```python
from build123d import *

# Parameters (mm, degrees)
SKETCH1_R           = 25.4
SKETCH1_R_2         = 19.05
BOSS_EXTRUDE1_DEPTH = 50.8
SKETCH4_R           = 25.4
SKETCH4_R_2         = 23.8125
CUT_EXTRUDE1_DEPTH  = 1.5875
FILLET1_R           = 0.762


with BuildPart() as part:
    # Sketch1 → Boss-Extrude1 (new body)
    with BuildSketch(Plane.XY):
        Circle(SKETCH1_R)
        Circle(SKETCH1_R_2, mode=Mode.SUBTRACT)
    extrude(amount=BOSS_EXTRUDE1_DEPTH)

    # Sketch4 → Cut-Extrude1 (cut)
    with BuildSketch(Plane(origin=(0, 0, 0), x_dir=(-1, 0, 0), z_dir=(0, 0, -1))):
        Circle(SKETCH4_R)
        Circle(SKETCH4_R_2, mode=Mode.SUBTRACT)
    cut_extrude1 = extrude(amount=-CUT_EXTRUDE1_DEPTH, mode=Mode.SUBTRACT)

    # Mirror1: Cut-Extrude1 across plane
    add(cut_extrude1.mirror(Plane.XY.offset(25.4)), mode=Mode.SUBTRACT)

    # Fillet1
    fillet1_edges = [part.edges().sort_by_distance(p)[0] for p in [
        (23.8125, 0, 1.5875),
        (23.8125, 0, 49.2125),
    ]]
    fillet(fillet1_edges, radius=FILLET1_R)


solid = part.part
```
Verification items for the finished model (mm, model axes). A direction names the side the tool comes from. Round coordinates to 2 decimals unless told otherwise and drop trailing zeros. Write each loop counter-clockwise with the first axis right and the second up, starting at its lowest first coordinate (ties: lowest second). Pieces come first, ordered by that corner, then holes. Notation, with made-up numbers: (-23, -0.75) -> (24, -0.75) arc R19 cw to (24, 10.25) -> close; hole circle Ø5 at (11.25, -28). An arc over 180 degrees is marked (long way). Write each question's results on one line, items separated by ' | '.
Q1. Go/stop test with flat-tipped pins: pin 1 Ø12 at (x, z) = (15.5, 13) entering from -Y; pin 2 Ø4 at (y, z) = (9, 24) entering from +X; pin 3 Ø1.5 at (y, z) = (-11.5, 18.5) entering from +X; pin 4 Ø12 at (x, y) = (-7, 3.5) entering from +Z. Record where each tip stops, or that it passes through.
Derived:
pin 1: stops at y = -23.56 | pin 2: stops at x = 24.42 | pin 3: stops at x = 23.01 | pin 4: passes through
Q2. Thickness scan on probe 1 along Y at (x, z) = (0, 39); probe 2 along Y at (x, z) = (-13.5, 47.5); probe 3 along X at (y, z) = (10, 5). Record the ranges inside material, lowest first.
Derived:
probe 1: y = -25.4 to -19.05, 19.05 to 25.4 | probe 2: y = -21.52 to -13.44, 13.44 to 21.52 | probe 3: x = -23.35 to -16.21, 16.21 to 23.35
Q3. Sectioned sample at C-C, the plane z = 28. Record the boundary of the cut face in (x, y), and give its area (3 significant figures).
Derived:
outline: circle Ø50.8 at (0, 0); hole circle Ø38.1 at (0, 0) | area: 887 mm²
Q4. Access from +Z, -Z, +X, -X, +Y, -Y to the whole of each face (thin tool, end or side, straight path). Record for faces 1 (the face through (-11, 16, 0)), 2 (the face through (18.897, -14.49, 50.393)), 3 (the face through (10, 23, 1.588)).
Derived:
face 1: -Z, +X, -X, +Y, -Y | face 2: +Z | face 3: -Z
Q5. Sectioned sample at A-A, the plane y = 0. Record the boundary of the cut face in (x, z), and give its area (3 significant figures).
Derived:
outline: (-25.4, 1.59) -> (-24.57, 1.59) arc R0.76 cw to (-23.81, 0.83) -> (-23.81, 0) -> (-19.05, 0) -> (-19.05, 50.8) -> (-23.81, 50.8) -> (-23.81, 49.97) arc R0.76 cw to (-24.57, 49.21) -> (-25.4, 49.21) -> close; (19.05, 0) -> (23.81, 0) -> (23.81, 0.83) arc R0.76 cw to (24.57, 1.59) -> (25.4, 1.59) -> (25.4, 49.21) -> (24.57, 49.21) arc R0.76 cw to (23.81, 49.97) -> (23.81, 50.8) -> (19.05, 50.8) -> close | area: 636 mm²
Q6. Draft check along Y on faces 4 (the face through (10, 23, 49.212)), 5 (the face through (-5.506, -24.796, 25.067)), 6 (the face through (-15.12, -11.59, 25.04)). Enter one of: released by +Y, released by -Y, zero draft, split by the parting line, or undercut.
Derived:
face 4: zero draft | face 5: split by the parting line | face 6: undercut
